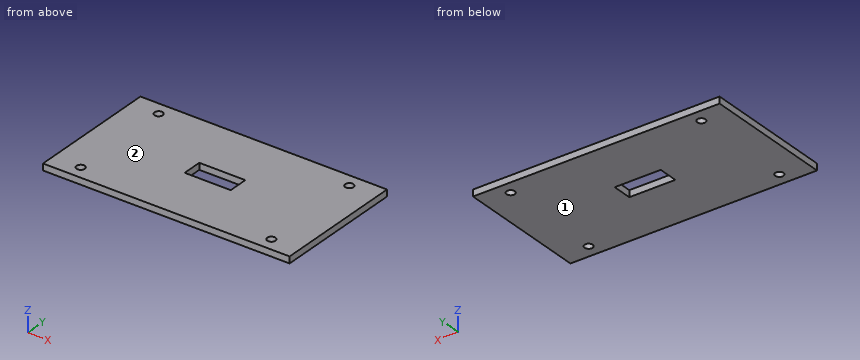
from build123d import *

# Parameters (mm, degrees)
ESBO_O1_W                = 150
ESBO_O1_H                = 80
ESBO_O1_R                = 2.5
ESBO_O1_W_2              = 28
ESBO_O1_H_2              = 12
RESSALTO_EXTRUS_O2_DEPTH = 4


with BuildPart() as part:
    # Esboço1 → Ressalto-extrusão2 (new body)
    with BuildSketch(Plane.XY):
        with Locations((25.444262425, 7.949915335)):
            Rectangle(ESBO_O1_W, ESBO_O1_H)
        with Locations((-32.555737575, 39.949915335)):
            Circle(ESBO_O1_R, mode=Mode.SUBTRACT)
        with Locations((-32.555737575, -24.050084665)):
            Circle(ESBO_O1_R, mode=Mode.SUBTRACT)
        with Locations((83.444262425, 39.949915335)):
            Circle(ESBO_O1_R, mode=Mode.SUBTRACT)
        with Locations((83.444262425, -24.050084665)):
            Circle(ESBO_O1_R, mode=Mode.SUBTRACT)
        with Locations((25.444262425, 7.949915335)):
            Rectangle(ESBO_O1_W_2, ESBO_O1_H_2, mode=Mode.SUBTRACT)
    extrude(amount=RESSALTO_EXTRUS_O2_DEPTH)


solid = part.part
The model under review builds one solid part; all positions refer to its coordinate system, in mm. Face numbers are marked on the shaded views. Give positions to 0.01 mm unless a question says otherwise; leave off trailing zeros. Order: outer loops, then holes, each group sorted by start corner. A loop starts at its lowest first (then second) coordinate and runs counter-clockwise, first axis right, second up. Notation, with made-up numbers: (22, 30.25) -> (78, 30.25) arc R12 cw to (78, 48.25) -> close; hole circle Ø8 at (62.5, -20). An arc over 180 degrees is marked (long way). Write item = value, one per line. Start each with the question number.
(1) Draft analysis for pull direction Z (two halves, no side actions). For the marked faces 1 and 2, state which applies: +Z half, -Z half, draft (parallel to the pull), parting line (faces both ways), or undercut.
(2) For pin 1 Ø6.5 at (x, y) = (-32.56, -24.05) entering from +Z; pin 2 Ø4.5 at (x, y) = (-32.56, 39.95) entering from +Z, all flat-tipped, find the tip position at first contact; note any pin that passes through.
(3) Take a section at A-A (x = 25). Write out the cut boundary in (y, z).
(4) For L1, parallel to X at y = 7, z = 0.9; L2, parallel to Y at x = 16, z = 2.15; L3, parallel to X at y = -23, z = 0.75, list the stretches that pass through material, from the lowest coordinate up. Write a range as from..to.
(5) Take a section at B-B (z = 1.85). Write out the cut boundary in (x, y), plus the area to 3 significant figures.
Returned:
q1.face_1 = -Z half
q1.face_2 = +Z half
q2.pin_1 = 4
q2.pin_2 = through
q3.outline = (-32.05, 0) -> (1.95, 0) -> (1.95, 4) -> (-32.05, 4) -> close; (13.95, 0) -> (47.95, 0) -> (47.95, 4) -> (13.95, 4) -> close
q4.L1 = -49.56..11.44, 39.44..100.44
q4.L2 = -32.05..1.95, 13.95..47.95
q4.L3 = -49.56..-34.82, -30.29..81.18, 85.71..100.44
q5.outline = (-49.56, -32.05) -> (100.44, -32.05) -> (100.44, 47.95) -> (-49.56, 47.95) -> close; hole circle Ø5 at (-32.56, -24.05); hole circle Ø5 at (-32.56, 39.95); hole (11.44, 1.95) -> (39.44, 1.95) -> (39.44, 13.95) -> (11.44, 13.95) -> close; hole circle Ø5 at (83.44, -24.05); hole circle Ø5 at (83.44, 39.95)
q5.area = 11,600 mm²
